```python
from build123d import *

# Parameters (mm, degrees)
F0_W     = 63
F0_H     = 63
F1_DEPTH = 35
F2_T     = -3
F4_R     = 1
F5_DEPTH = 25


with BuildPart() as f1:
    # F0 (on Front) → F1 (new body)
    with BuildSketch(Plane.XZ):
        Rectangle(F0_W, F0_H)
    extrude(amount=F1_DEPTH)

    # F2
    f2_openings = [f1.faces().sort_by_distance(p)[0] for p in [
        (0, -35, 0),
    ]]
    offset(amount=F2_T, openings=f2_openings)

    # F4 (on Front) → F5 (cut)
    with BuildSketch(Plane.XZ):
        with Locations((7.88837, 0)):
            Circle(F4_R)
        with Locations((-7.888372, 0)):
            Circle(F4_R)
        with Locations((0, 7.88837)):
            Circle(F4_R)
        with Locations((0, -7.88837)):
            Circle(F4_R)
        Circle(F4_R)
    extrude(amount=F5_DEPTH, mode=Mode.SUBTRACT)


solid = f1.part
```
Read the model definition and answer for the solid it produces. Units are mm, in the model's axes. A direction names the side the tool comes from. Round coordinates to 2 decimals unless told otherwise and drop trailing zeros. Write each loop counter-clockwise with the first axis right and the second up, starting at its lowest first coordinate (ties: lowest second). Pieces come first, ordered by that corner, then holes. Notation, with made-up numbers: (-15, -7) -> (29, -7) arc R23 ccw to (29, 20) -> close; hole circle Ø8 at (-6, 50.25). An arc over 180 degrees is marked (long way). Answer in a Markdown table with one row per item. Add a question column.
1) Find section B-B, the plane z = 0. Determine the outline of the cut face in (x, y), and give its area (3 significant figures).
2) Find section A-A, the plane x = 0. Determine the outline of the cut face in (y, z).
3) Consider line 1 (Z direction, x = -12, y = -20.5); line 2 (Y direction, x = 28, z = 2). Determine where each line is inside the solid, lowest interval first.
4) Find section D-D, the plane z = 15. Determine the outline of the cut face in (x, y), and give its area (3 significant figures).
5) Given P1, Ø1.6, axis at x = -7.89, z = 0, coming from the +Y side; P2, Ø2.5, axis at x = 0, z = -7.89, coming from the +Y side; P3, Ø2.5, axis at x = 7.89, z = 0, coming from the -Y side, each flat-ended and moving along its own axis, determine where each tip first touches the part or whether it passes through.
6) Find section C-C, the plane y = -13. Determine the outline of the cut face in (x, z).
7) Which of the six approach directions +Z, -Z, +X, -X, +Y, -Y give full straight-line access (tool end or side, diameter ignored) to faces 5 (the face through (0, -17, 31.5)), 6 (the face through (0, -19, 28.5))?
8) Determine the mould class of faces 1 (the face through (-2, -35, -30)), 2 (the face through (0, -17, -31.5)), 3 (the face through (-0.13, -1.48, 8.88)), 4 (the face through (6.89, -1.48, 0.04)) for opening direction Z: pulls with the +Z half, pulls with the -Z half, needs draft (parallel to the pull), parting line crosses it, or undercut.
Findings below:
| question | item | result |
|---|---|---|
| 1 | outline | (-31.5, -35) -> (-28.5, -35) -> (-28.5, -3) -> (-8.89, -3) -> (-8.89, 0) -> (-31.5, 0) -> close; (-6.89, -3) -> (-1, -3) -> (-1, 0) -> (-6.89, 0) -> close; (1, -3) -> (6.89, -3) -> (6.89, 0) -> (1, 0) -> close; (8.89, -3) -> (28.5, -3) -> (28.5, -35) -> (31.5, -35) -> (31.5, 0) -> (8.89, 0) -> close |
| 1 | area | 363 mm² |
| 2 | outline | (-35, -31.5) -> (0, -31.5) -> (0, -8.89) -> (-3, -8.89) -> (-3, -28.5) -> (-35, -28.5) -> close; (-35, 28.5) -> (-3, 28.5) -> (-3, 8.89) -> (0, 8.89) -> (0, 31.5) -> (-35, 31.5) -> close; (-3, -6.89) -> (0, -6.89) -> (0, -1) -> (-3, -1) -> close; (-3, 1) -> (0, 1) -> (0, 6.89) -> (-3, 6.89) -> close |
| 3 | line 1 | -31.5 to -28.5, 28.5 to 31.5 |
| 3 | line 2 | -3 to 0 |
| 4 | outline | (-31.5, -35) -> (-28.5, -35) -> (-28.5, -3) -> (28.5, -3) -> (28.5, -35) -> (31.5, -35) -> (31.5, 0) -> (-31.5, 0) -> close |
| 4 | area | 381 mm² |
| 5 | P1 | through |
| 5 | P2 | y = 0 |
| 5 | P3 | y = -3 |
| 6 | outline | (-31.5, -31.5) -> (31.5, -31.5) -> (31.5, 31.5) -> (-31.5, 31.5) -> close; hole (-28.5, -28.5) -> (28.5, -28.5) -> (28.5, 28.5) -> (-28.5, 28.5) -> close |
| 7 | face 5 | +Z, +X, -X, +Y, -Y |
| 7 | face 6 | -Y |
| 8 | face 1 | needs draft |
| 8 | face 2 | pulls with the -Z half |
| 8 | face 3 | undercut |
| 8 | face 4 | undercut |
